from build123d import *

# Parameters (mm, degrees)
SKETCH1_R           = 40.538
SKETCH1_R_2         = 27.506
BOSS_EXTRUDE1_DEPTH = 1
SKETCH4_R           = 10.65
CUT_EXTRUDE1_DEPTH  = 1


with BuildPart() as part:
    # Sketch1 → Boss-Extrude1 (new body)
    with BuildSketch(Plane(origin=(0, 0, 0), x_dir=(-1, 0, 0), z_dir=(0, 1, 0))):
        with Locations(Location((-29.391570254, 2.611368154, 0), (0, 0, 90))):
            Circle(SKETCH1_R)
        with Locations(Location((-29.391570254, 2.611368154, 0), (0, 0, 90))):
            Circle(SKETCH1_R_2, mode=Mode.SUBTRACT)
    extrude(amount=BOSS_EXTRUDE1_DEPTH)

    # Sketch4 → Cut-Extrude1 (cut)
    with BuildSketch(Plane.XZ):
        with Locations((4.223815401, 32.628524909)):
            Circle(SKETCH4_R)
        with Locations((54.559325107, 32.628524909)):
            Circle(SKETCH4_R)
        with Locations((63.829694025, -16.055747722)):
            Circle(SKETCH4_R)
        with Locations((-5.046553517, -16.055747722)):
            Circle(SKETCH4_R)
    extrude(amount=-CUT_EXTRUDE1_DEPTH, mode=Mode.SUBTRACT)


solid = part.part
Here's how the part is built. I have some questions about the finished solid (model axes, mm). Round coordinates to 2 decimals unless told otherwise and drop trailing zeros. Order: outer loops, then holes, each group sorted by start corner. A loop starts at its lowest first (then second) coordinate and runs counter-clockwise, first axis right, second up. Notation, with made-up numbers: (-36.75, 38) -> (-32.75, 38) arc R30 ccw to (-32.75, 62) -> close; hole circle Ø11 at (56, -35). An arc over 180 degrees is marked (long way). Return JSON: item names as keys, results as strings.
Q1. If we section it at B-B on z = -3: List the corners of the cut face in (x, y) for me, plus the area to 3 significant figures.
Filled sheet:
{"outline": "(-10.76, 0) -> (2.46, 0) -> (2.46, 1) -> (-10.76, 1) -> close; (56.32, 0) -> (69.54, 0) -> (69.54, 1) -> (56.32, 1) -> close", "area": "26.4 mm^2"}
Q2. If we section it at A-A on x = 55: List the corners of the cut face in (y, z) for me.
Filled sheet:
{"outline": "(0, -28.81) -> (1, -28.81) -> (1, -22.01) -> (0, -22.01) -> close; (0, -10.1) -> (1, -10.1) -> (1, -7.43) -> (0, -7.43) -> close; (0, 12.65) -> (1, 12.65) -> (1, 21.99) -> (0, 21.99) -> close"}
Q3. I need wall thicknesses on line 1 along Z through (x, y) = (54, 0.4); line 2 along X through (y, z) = (0.9, 18); line 3 along Z through (x, y) = (32, 0.15). Which ranges of each line are inside material? Lowest first, please. Write a range as from..to.
Filled sheet:
{"line 1": "z = -29.6..-20.15, -11.96..-9.68, 14.9..21.99", "line 2": "x = -8.11..6.59, 52.19..66.9", "line 3": "z = -37.84..-24.77, 29.99..43.07"}
Q4. If we section it at C-C on y = 0.8: List the corners of the cut face in (x, z) for me.
Filled sheet:
{"outline": "(-10.07, -6.67) arc R10.65 cw to (0.08, -25.39) arc R40.54 ccw to (58.7, -25.39) arc R10.65 cw to (68.85, -6.67) arc R40.54 ccw to (62.68, 25.74) arc R10.65 cw to (46.36, 39.43) arc R40.54 ccw to (12.42, 39.43) arc R10.65 cw to (-3.9, 25.74) arc R40.54 ccw to start; hole circle Ø55.01 at (29.39, 2.61)"}
Q5. If we mould it in two halves opening along X, with no side actions, what happens to faces 1 (the cylindrical face through (52.585, 0.493, 17.398)), 2 (the flat face through (36, 1, -25)), 3 (the cylindrical face through (-10.475, 0.493, 9.961))? For each: released by +X, released by -X, zero draft, split by the parting line, or undercut.
Filled sheet:
{"face 1": "undercut", "face 2": "zero draft", "face 3": "released by -X"}
Q6. If we section it at D-D on x = 25: List the corners of the cut face in (y, z) for me.
Filled sheet:
{"outline": "(0, -37.69) -> (1, -37.69) -> (1, -24.54) -> (0, -24.54) -> close; (0, 29.76) -> (1, 29.76) -> (1, 42.91) -> (0, 42.91) -> close"}
